Here's how the part is built. I have some questions about the finished solid (model axes, mm). A direction names the side the tool comes from. Coordinates: 2 decimals unless noted, no trailing zeros. Write each loop counter-clockwise with the first axis right and the second up, starting at its lowest first coordinate (ties: lowest second). Pieces come first, ordered by that corner, then holes. Notation, with made-up numbers: (72, 68.5) -> (78, 68.5) arc R23 ccw to (78, 78.5) -> close; hole circle Ø10 at (40, 60.25). An arc over 180 degrees is marked (long way). Use a Markdown table: item, result. Add a question column.
```python
from build123d import *

# Parameters (mm, degrees)
F0_W     = 64
F0_H     = 45
F1_DEPTH = 10


with BuildPart() as f1:
    # F0 (on Top) → F1 (new body)
    with BuildSketch(Plane.XY):
        Rectangle(F0_W, F0_H)
        with BuildLine():
            ThreePointArc((15.282927, 4.053659), (0, -3), (-15.282927, 4.053659))
            Line((-15.282927, 4.053659), (-15.282927, 7.053659))
            ThreePointArc((-15.282927, 7.053659), (0, 0), (15.282927, 7.053659))
            Line((15.282927, 7.053659), (15.282927, 4.053659))
        make_face(mode=Mode.SUBTRACT)
    extrude(amount=F1_DEPTH)


solid = f1.part
```
Q1. Will this pin go through, and if not, where does the flat tip stop? pin 1 (3 mm diameter, centred on x = -13.5, y = 9.5, fed in from -Z).
Q2. Suppose I cut it at A-A, the plane z = 6.25. Write out the boundary of the cut face in (x, y).
Q3. Please list where these lines run through material, in increasing order: line 1 (X direction, y = 3, z = 8); line 2 (X direction, y = 5, z = 5.75); line 3 (Y direction, x = 13.5, z = 1).
Q4. Suppose I cut it at B-B, the plane y = 1.5. Write out the boundary of the cut face in (x, z), and give its area (3 significant figures).
Q5. Thinking about a two-plate mould opening in X: for faces 1 (the flat face through (-32, 0, 5)), 2 (the flat face through (32, 0, 5)), 3 (the flat face through (15.283, 6, 5)), 4 (the flat face through (0, 22.5, 5)), which applies, released by +X, released by -X, zero draft, split by the parting line, or undercut?
Q6. Suppose I cut it at C-C, the plane x = 14.5. Write out the boundary of the cut face in (y, z), and give its area (3 significant figures).
Q7. Which directions (+Z, -Z, +X, -X, +Y, -Y) give clear straight access to the entire face, cutting with the end or side of a thin tool? Please do faces 5 (the flat face through (-0.4, 0.3, 10)), 6 (the cylindrical face through (0, -3, 5)).
Answer key:
| question | item | result |
|---|---|---|
| 1 | pin 1 | stops at z = 0 |
| 2 | outline | (-32, -22.5) -> (32, -22.5) -> (32, 22.5) -> (-32, 22.5) -> close; hole (-15.28, 4.05) arc R20.08 ccw to (15.28, 4.05) -> (15.28, 7.05) arc R20.08 cw to (-15.28, 7.05) -> close |
| 3 | line 1 | x = -32 to -14.32, -10.56 to 10.56, 14.32 to 32 |
| 3 | line 2 | x = -32 to -15.28, -13.26 to 13.26, 15.28 to 32 |
| 3 | line 3 | y = -22.5 to 2.21, 5.21 to 22.5 |
| 4 | outline | (-32, 0) -> (-12.67, 0) -> (-12.67, 10) -> (-32, 10) -> close; (-7.62, 0) -> (7.62, 0) -> (7.62, 10) -> (-7.62, 10) -> close; (12.67, 0) -> (32, 0) -> (32, 10) -> (12.67, 10) -> close |
| 4 | area | 539 mm^2 |
| 5 | face 1 | released by -X |
| 5 | face 2 | released by +X |
| 5 | face 3 | undercut |
| 5 | face 4 | zero draft |
| 6 | outline | (-22.5, 0) -> (3.19, 0) -> (3.19, 10) -> (-22.5, 10) -> close; (6.19, 0) -> (22.5, 0) -> (22.5, 10) -> (6.19, 10) -> close |
| 6 | area | 420 mm^2 |
| 7 | face 5 | +Z, +X, -X, +Y, -Y |
| 7 | face 6 | +Z, -Z |
